from build123d import *

# Parameters (mm, degrees)
F0_R     = 15.875
F1_DEPTH = 3.175
F2_DEPTH = 19.05
F3_R     = 15.875
F4_DEPTH = 3.175


with BuildPart() as f1:
    # F0 (on Top) → F1 (new body)
    with BuildSketch(Plane.XY):
        with BuildLine():
            ThreePointArc((101.6, 0), (-7.961986, 101.287545), (-100.352102, -15.875))
            Line((-100.352102, -15.875), (100.352102, -15.875))
            ThreePointArc((100.352102, -15.875), (101.287545, -7.961986), (101.6, 0))
        make_face()
        with Locations((0, 6.35)):
            Circle(F0_R, mode=Mode.SUBTRACT)
    extrude(amount=F1_DEPTH)

    # F0 (on Top) → F2 (join)
    with BuildSketch(Plane.XY):
        with BuildLine():
            ThreePointArc((103.565366, -15.875), (104.472154, -7.960509), (104.775, 0))
            ThreePointArc((104.775, 0), (-7.960509, 104.472154), (-103.565366, -15.875))
            Line((-103.565366, -15.875), (-100.352102, -15.875))
            ThreePointArc((-100.352102, -15.875), (-7.961986, 101.287545), (101.6, 0))
            ThreePointArc((101.6, 0), (101.287545, -7.961986), (100.352102, -15.875))
            Line((100.352102, -15.875), (103.565366, -15.875))
        make_face()
    extrude(amount=F2_DEPTH)

    # F3 (on face) → F4 (join)
    with BuildSketch(Plane.XY.offset(19.05)):
        with BuildLine():
            ThreePointArc((103.565366, -15.875), (104.472154, -7.960509), (104.775, 0))
            ThreePointArc((104.775, 0), (-7.960509, 104.472154), (-103.565366, -15.875))
            Line((-103.565366, -15.875), (-100.352102, -15.875))
            Line((-100.352102, -15.875), (103.565366, -15.875))
        make_face()
        with Locations((0, 6.35)):
            Circle(F3_R, mode=Mode.SUBTRACT)
    extrude(amount=F4_DEPTH)


solid = f1.part
Here's how the part is built. I have some questions about the finished solid (model axes, mm). Round coordinates to 2 decimals unless told otherwise and drop trailing zeros. Loops run counter-clockwise (first coordinate to the right, second up) from the corner with the lowest first, then second, coordinate; pieces in that order, holes last. Notation, with made-up numbers: (32.5, 9.5) -> (47.5, 9.5) arc R16 ccw to (47.5, 15.5) -> close; hole circle Ø3 at (52, 15). An arc over 180 degrees is marked (long way). Write each question's results on one line, items separated by ' | '.
(1) If we section it at A-A, the plane x = 0: List the corners of the cut face in (y, z) for me (3 decimals), then the cut area to 3 significant figures.
Worked answers:
outline: (-15.875, 0) -> (-9.525, 0) -> (-9.525, 3.175) -> (-15.875, 3.175) -> close; (-15.875, 19.05) -> (-9.525, 19.05) -> (-9.525, 22.225) -> (-15.875, 22.225) -> close; (22.225, 0) -> (104.775, 0) -> (104.775, 22.225) -> (22.225, 22.225) -> (22.225, 19.05) -> (101.6, 19.05) -> (101.6, 3.175) -> (22.225, 3.175) -> close | area: 615 mm2
(2) We'd pull the mould along Y, two halves only. Please class faces 1 (the face through (-1, 32, 22.225)), 2 (the face through (101.296, -7.851, 11.001)), 3 (the face through (0, -15.875, 3)): released by +Y, released by -Y, zero draft, split by the parting line, or undercut.
Worked answers:
face 1: zero draft | face 2: undercut | face 3: released by -Y
(3) If we section it at B-B, the plane y = 38: List the corners of the cut face in (x, z) for me (3 decimals).
Worked answers:
outline: (-97.641, 0) -> (97.641, 0) -> (97.641, 22.225) -> (-97.641, 22.225) -> close; hole (-94.226, 3.175) -> (94.226, 3.175) -> (94.226, 19.05) -> (-94.226, 19.05) -> close
(4) If we section it at C-C, the plane y = 6.35: List the corners of the cut face in (x, z) for me (3 decimals), then the cut area to 3 significant figures.
Worked answers:
outline: (-104.582, 0) -> (-15.875, 0) -> (-15.875, 3.175) -> (-101.401, 3.175) -> (-101.401, 19.05) -> (-15.875, 19.05) -> (-15.875, 22.225) -> (-104.582, 22.225) -> close; (15.875, 0) -> (104.582, 0) -> (104.582, 22.225) -> (15.875, 22.225) -> (15.875, 19.05) -> (101.401, 19.05) -> (101.401, 3.175) -> (15.875, 3.175) -> close | area: 1,230 mm2
(5) If I drill on L1, parallel to Z at x = 10, y = 20 (3 decimals); L2, parallel to Y at x = 0, z = 20.95 (3 decimals); L3, parallel to X at y = 48, z = 11.5, over which ranges is the centre line in solid material (lowest first)?
Worked answers:
L1: 0 to 3.175, 19.05 to 22.225 | L2: -15.875 to -9.525, 22.225 to 104.775 | L3: -93.13 to -89.55, 89.55 to 93.13
(6) For P1, Ø6, axis at y = 24.5, z = 5.5, coming from the -X side; P2, Ø8, axis at x = 27.5, z = 11.5, coming from the -Y side; P3, Ø12, axis at x = 34.5, y = -1.5, coming from the -Z side; P4, Ø5, axis at x = 54.5, z = 11, coming from the +Y side, each with a flat end and sliding along its axis, tell me the tip position at first contact or that it passes through.
Worked answers:
P1: x = -102.55 | P2: y = 96.59 | P3: z = 0 | P4: y = 90.96
(7) If we section it at D-D, the plane z = 16: List the corners of the cut face in (x, y) for me (3 decimals), then the cut area to 3 significant figures.
Worked answers:
outline: (-103.565, -15.875) -> (-100.352, -15.875) arc R101.6 cw (long way) to (101.6, 0) arc R101.6 cw to (100.352, -15.875) -> (103.565, -15.875) arc R104.775 ccw to (104.775, 0) arc R104.775 ccw (long way) to start | area: 1,130 mm2
